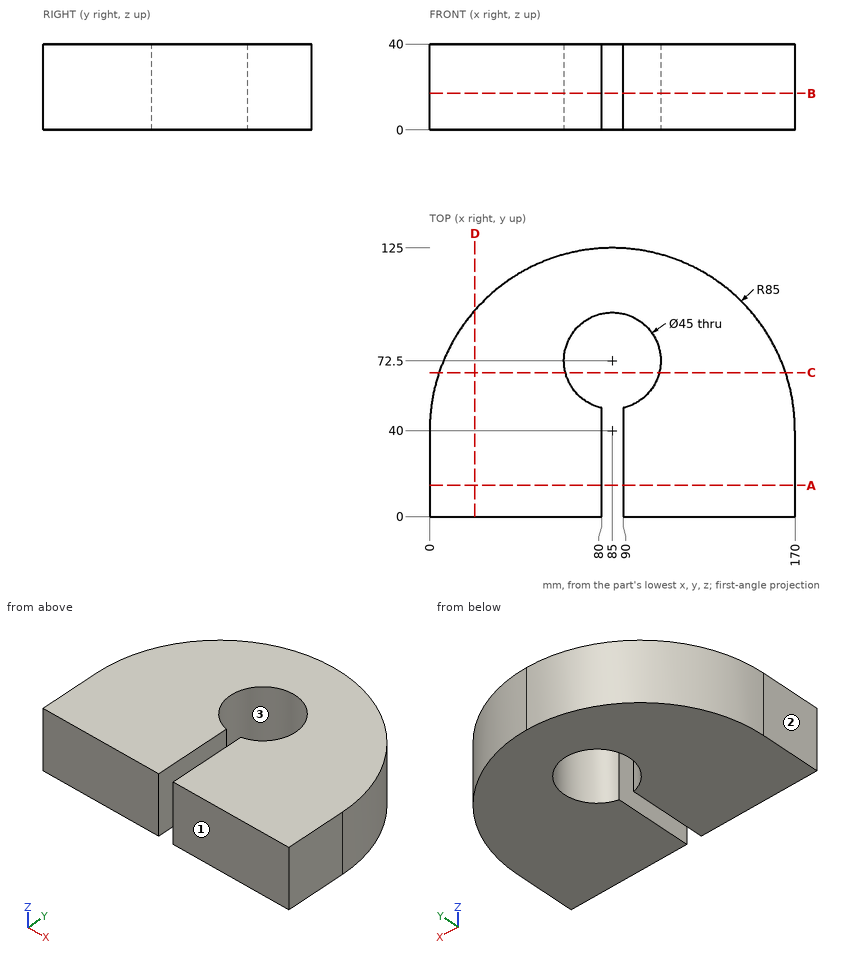
For this review, use the dimensioned drawing (mm, ordinates from the lowest corner) and the shaded views. Give positions to 0.01 mm unless a question says otherwise; leave off trailing zeros. Order: outer loops, then holes, each group sorted by start corner. A loop starts at its lowest first (then second) coordinate and runs counter-clockwise, first axis right, second up.
1) Take a section at A-A (y = 14.5). Give the boundary of the cut face in (x, z), then the cut area to 3 significant figures.
2) Take a section at D-D (x = 21). Give the boundary of the cut face in (y, z), then the cut area to 3 significant figures.
3) Take a section at C-C (y = 67). Give the boundary of the cut face in (x, z).
4) Insertion check: pin 1 (2 mm diameter, centred on y = 73.5, z = 10, fed in from -X); pin 2 (8 mm diameter, centred on y = 48.5, z = 6, fed in from -X); pin 3 (8 mm diameter, centred on y = 111.5, z = 32.5, fed in from -X). Each pin has a flat end and moves straight along its axis. Give the tip position at first contact, or say it passes through.
5) Wall thickness on line 1 (X direction, y = 32.5, z = 8.5); line 2 (X direction, y = 72.5, z = 20); line 3 (Y direction, x = 102, z = 33.5): over which ranges is each line inside the solid? List them lowest first.
6) Take a section at B-B (z = 17). Give the boundary of the cut face in (x, y).
7) The part is to be moulded in two halves that separate along Y. For the marked faces 1, 2 and 3, say which applies: released by +Y, released by -Y, zero draft, split by the parting line, or undercut.
Derived:
1. outline: (0, 0) - (80, 0) - (80, 40) - (0, 40) - close; (90, 0) - (170, 0) - (170, 40) - (90, 40) - close
1. area: 6,400 mm2
2. outline: (0, 0) - (95.94, 0) - (95.94, 40) - (0, 40) - close
2. area: 3,840 mm2
3. outline: (4.4, 0) - (63.18, 0) - (63.18, 40) - (4.4, 40) - close; (106.82, 0) - (165.6, 0) - (165.6, 40) - (106.82, 40) - close
4. pin 1: stops at x = 6.46
4. pin 2: stops at x = 0.12
4. pin 3: stops at x = 33.34
5. line 1: x = 0 to 80, 90 to 170
5. line 2: x = 6.46 to 62.5, 107.5 to 163.54
5. line 3: y = 0 to 57.76, 87.24 to 123.28
6. outline: (0, 0) - (80, 0) - (80, 50.56) arc R22.5 cw (long way) to (90, 50.56) - (90, 0) - (170, 0) - (170, 40) arc R85 ccw to (85, 125) arc R85 ccw to (0, 40) - close
7. face 1: released by -Y
7. face 2: zero draft
7. face 3: undercut
